```python
from build123d import *

# Parameters (mm, degrees)
PAD003_DEPTH = 3.5
POCKET_DEPTH = 5.5
SKETCH011_W  = 5
SKETCH011_H  = 7.2


with BuildPart() as obj1:
    # Sketch010 → Pad003 (new body, symmetric)
    with BuildSketch(Plane.XY):
        with BuildLine():
            ThreePointArc((59.498979, 20.271308), (30.157918, 27.585958), (0, 29.8))
            Line((0, 29.8), (0, 16.6))
            ThreePointArc((58.317055, 0.623642), (30.232941, 12.533656), (0, 16.6))
            ThreePointArc((58.317055, 0.623642), (63.354776, 0.781276), (65.351677, 5.409004))
            Line((63.7883, 15.177117), (65.351677, 5.409004))
            ThreePointArc((63.7883, 15.177117), (62.350118, 18.319069), (59.498979, 20.271308))
        make_face()
    extrude(amount=PAD003_DEPTH, both=True)

    # Sketch009 → Pocket (cut)
    with BuildSketch(Plane.XY.offset(3.5)):
        with BuildLine():
            Line((0, 27.898268), (0, 18.183007))
            ThreePointArc((57.375322, 3.010124), (29.674349, 14.327664), (0, 18.183007))
            ThreePointArc((57.375322, 3.010124), (58.546948, 3.277627), (58.382807, 4.46814))
            ThreePointArc((58.112759, 15.405314), (55.75963, 9.875292), (58.382807, 4.46814))
            ThreePointArc((58.112759, 15.405314), (58.750082, 17.397997), (57.35497, 18.957045))
            ThreePointArc((57.35497, 18.957045), (29.050369, 25.819583), (0, 27.898268))
        make_face()
    extrude(amount=-POCKET_DEPTH, mode=Mode.SUBTRACT)

    # Sketch011 (on Face2 of Pocket) → Groove (revolve, cut)
    with BuildSketch(Plane(origin=(62.588677, 10.017255, 0), x_dir=(-0.158038, 0.987433, 0), z_dir=(0.987433, 0.158038, 0))):
        with Locations((2.5, 0)):
            Rectangle(SKETCH011_W, SKETCH011_H)
    revolve(axis=Axis((62.588677, 10.017255, 0), (0, 0, 1)), mode=Mode.SUBTRACT)


with BuildPart() as part_mirroring:
    # Part__Mirroring: instance of obj1
    add(obj1.part.mirror(Plane(origin=(0, 0, 0), x_dir=(0, -1, 0), z_dir=(1, 0, 0))))


solid = part_mirroring.part
```
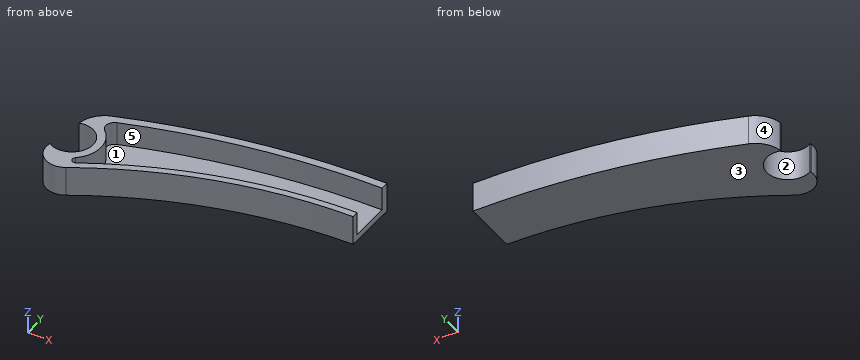
Can you work these out from the model? Positions are in its coordinate system, mm. Face numbers are marked on the shaded views. A direction names the side the tool comes from. Round coordinates to 2 decimals unless told otherwise and drop trailing zeros. Loops run counter-clockwise (first coordinate to the right, second up) from the corner with the lowest first, then second, coordinate; pieces in that order, holes last.
Item 1: Please list where these lines run through material, in increasing order: L1, parallel to Z at x = -27.5, y = 16; L2, parallel to Y at x = -17, z = 1.75; L3, parallel to Y at x = -21, z = -1.
Item 2: Suppose I cut it at B-B, the plane y = 11.25. Write out the boundary of the cut face in (x, z), then the cut area to 3 significant figures.
Item 3: Will these pins go through, and if not, where does the flat tip stop? pin 1 Ø4 at (x, z) = (-13, 3) entering from +Y; pin 2 Ø2 at (x, z) = (-41, 0.5) entering from +Y; pin 3 Ø4 at (x, z) = (-23.5, 2.5) entering from -Y.
Item 4: Suppose I cut it at A-A, the plane z = -2.75. Write out the boundary of the cut face in (x, y).
Item 5: If we mould it in two halves opening along Y, with no side actions, what happens to the marked faces 3, 4 and 5? For each: +Y half, -Y half, draft (parallel to the pull), parting line (faces both ways), or undercut.
Item 6: Which directions (+Z, -Z, +X, -X, +Y, -Y) give clear straight access to the entire face, cutting with the end or side of a thin tool? Please do the marked faces 1 and 2.
Reported:
1. L1: z = -3.5 to -2
1. L2: y = 15.33 to 16.93, 27.27 to 29.19
1. L3: y = 14.66 to 16.27, 26.88 to 28.81
2. outline: (-57.74, -3.5) - (-34.58, -3.5) - (-34.58, 3.5) - (-39.52, 3.5) - (-39.52, -2) - (-55.86, -2) - (-55.86, 3.5) - (-57.74, 3.5) - close
2. area: 72.3 mm2
3. pin 1: stops at y = 29.59
3. pin 2: stops at y = 25.72
3. pin 3: stops at y = 13.72
4. outline: (-65.35, 5.41) arc R4.7 ccw to (-58.32, 0.62) arc R114.42 cw to (0, 16.6) - (0, 29.8) arc R177.02 ccw to (-59.5, 20.27) arc R6.46 ccw to (-63.79, 15.18) - (-63.84, 14.86) arc R5 cw (long way) to (-65.29, 5.81) - close
5. face 3: draft
5. face 4: +Y half
5. face 5: undercut
6. face 1: +Z
6. face 2: +Z, -Z
